```python
from build123d import *

# Parameters (mm, degrees)
SKETCH1_W           = 100
SKETCH1_H           = 30
SKETCH1_R           = 9.5
SKETCH1_R_2         = 1.5
BOSS_EXTRUDE1_DEPTH = 2
SKETCH2_W           = 100
SKETCH2_H           = 30
SKETCH2_W_2         = 96
SKETCH2_H_2         = 26
BOSS_EXTRUDE3_DEPTH = 50
CUT_EXTRUDE1_REACH  = 102
SKETCH4_R           = 5
SKETCH5_R           = 1.5
CUT_EXTRUDE2_DEPTH  = 101
SKETCH6_R           = 3
CUT_EXTRUDE3_DEPTH  = 101


with BuildPart() as part:
    # Sketch1 → Boss-Extrude1 (new body)
    with BuildSketch(Plane.XY):
        Rectangle(SKETCH1_W, SKETCH1_H)
        with Locations((-25, -3)):
            Circle(SKETCH1_R, mode=Mode.SUBTRACT)
        with Locations((-40, -3)):
            Circle(SKETCH1_R_2, mode=Mode.SUBTRACT)
        with Locations((-32.5, 9.990381057)):
            Circle(SKETCH1_R_2, mode=Mode.SUBTRACT)
        with Locations((-17.5, 9.990381057)):
            Circle(SKETCH1_R_2, mode=Mode.SUBTRACT)
        with Locations((-10, -3)):
            Circle(SKETCH1_R_2, mode=Mode.SUBTRACT)
        with Locations((25, -3)):
            Circle(SKETCH1_R_2, mode=Mode.SUBTRACT)
    extrude(amount=BOSS_EXTRUDE1_DEPTH)

    # Sketch2 → Boss-Extrude3 (add)
    with BuildSketch(Plane.XY.offset(2)):
        Rectangle(SKETCH2_W, SKETCH2_H)
        Rectangle(SKETCH2_W_2, SKETCH2_H_2, mode=Mode.SUBTRACT)
    extrude(amount=-BOSS_EXTRUDE3_DEPTH)

    # Sketch4 → Cut-Extrude1 (cut, up to next)
    with BuildSketch(Plane.ZY.offset(50), mode=Mode.PRIVATE) as cut_extrude1_sk1:
        with Locations((-38, 3)):
            Circle(SKETCH4_R)
    cut_extrude1_tool1 = extrude(cut_extrude1_sk1.sketch, amount=-CUT_EXTRUDE1_REACH, mode=Mode.PRIVATE) & part.part
    add(cut_extrude1_tool1.solids().sort_by_distance((-50, 3, -38))[0], mode=Mode.SUBTRACT)

    # Sketch5 → Cut-Extrude2 (cut, through all)
    with BuildSketch(Plane.ZY.offset(50)):
        with Locations((-45, 10)):
            Circle(SKETCH5_R)
        with Locations((-45, -10)):
            Circle(SKETCH5_R)
    extrude(amount=-CUT_EXTRUDE2_DEPTH, mode=Mode.SUBTRACT)

    # Sketch6 → Cut-Extrude3 (cut, through all)
    with BuildSketch(Plane.ZY.offset(50)):
        with Locations((-23, -5)):
            Circle(SKETCH6_R)
    extrude(amount=-CUT_EXTRUDE3_DEPTH, mode=Mode.SUBTRACT)


solid = part.part
```
Work out the finished part from the listing and answer in its coordinate system (mm). A direction names the side the tool comes from. Coordinates: 2 decimals unless noted, no trailing zeros. Write each loop counter-clockwise with the first axis right and the second up, starting at its lowest first coordinate (ties: lowest second). Pieces come first, ordered by that corner, then holes.
Q1. A cutting plane is placed at B-B, the plane z = -17. Give the vertices of the cut face in (x, y), then the cut area to 3 significant figures.
Q2. A cutting plane is placed at C-C, the plane y = 3. Give the vertices of the cut face in (x, z), then the cut area to 3 significant figures.
Q3. A cutting plane is placed at A-A, the plane x = -25. Give the vertices of the cut face in (y, z).
Q4. Which of the six approach directions +Z, -Z, +X, -X, +Y, -Y give full straight-line access (tool end or side, diameter ignored) to faces 4 (the face through (-33.61, 11, 0.99)), 5 (the face through (-49, 3, -43)), 6 (the face through (-48, 0, -24))?
Q5. Determine the mould class of faces 1 (the face through (-50, 0, -23)), 2 (the face through (-49.01, 10.07, -46.5)), 3 (the face through (-1, 0, 2)) for opening direction Z: released by +Z, released by -Z, zero draft, split by the parting line, or undercut.
Q6. A cutting plane is placed at D-D, the plane y = -10. Give the vertices of the cut face in (x, z), then the cut area to 3 significant figures.
Q7. Find the intervals of material crossed by line 1 (Y direction, x = -49.35, z = -45); line 2 (Y direction, x = 49.25, z = -23); line 3 (Y direction, x = 29.5, z = -1), in increasing order.
Q8. Each of these flat-tipped pins is pushed along its axis until it touches: pin 1 Ø2.5 at (y, z) = (-10, -45) entering from +X; pin 2 Ø1 at (x, y) = (-5, 5.5) entering from -Z. Where does it stop, or does it pass through?
Findings below:
1. outline: (-50, -15) - (50, -15) - (50, 15) - (-50, 15) - close; hole (-48, -13) - (48, -13) - (48, 13) - (-48, 13) - close
1. area: 504 mm2
2. outline: (-50, -48) - (-48, -48) - (-48, -43) - (-50, -43) - close; (-50, -33) - (-48, -33) - (-48, 0) - (-32.37, 0) - (-32.37, 2) - (-50, 2) - close; (-17.63, 0) - (48, 0) - (48, -48) - (50, -48) - (50, 2) - (-17.63, 2) - close
2. area: 343 mm2
3. outline: (-15, -48) - (-13, -48) - (-13, 0) - (-12.5, 0) - (-12.5, 2) - (-15, 2) - close; (6.5, 0) - (13, 0) - (13, -48) - (15, -48) - (15, 2) - (6.5, 2) - close
4. face 4: +Z, -Z
4. face 5: -X
4. face 6: -Z
5. face 1: zero draft
5. face 2: undercut
5. face 3: released by +Z
6. outline: (-50, -48) - (-48, -48) - (-48, -46.5) - (-50, -46.5) - close; (-50, -43.5) - (-48, -43.5) - (-48, 0) - (-31.42, 0) - (-31.42, 2) - (-50, 2) - close; (-18.58, 0) - (48, 0) - (48, -43.5) - (50, -43.5) - (50, 2) - (-18.58, 2) - close; (48, -48) - (50, -48) - (50, -46.5) - (48, -46.5) - close
6. area: 354 mm2
7. line 1: y = -15 to -11.5, -8.5 to 8.5, 11.5 to 15
7. line 2: y = -15 to -8, -2 to 15
7. line 3: y = -15 to -13, 13 to 15
8. pin 1: passes through
8. pin 2: stops at z = 0
